```python
from build123d import *

# Parameters (mm, degrees)
SKETCH1_R                                       = 1.6
BASE_FLANGE1_DEPTH                              = 3
EDGE_FLANGE1_START                              = -44
EDGE_FLANGE1_DEPTH                              = 10.5
EDGE_FLANGE1_START_2                            = 33.5
EDGE_FLANGE1_2_DEPTH                            = 10.5
EDGE_FLANGE1_START_3                            = -35
EDGE_FLANGE1_3_DEPTH                            = 1.5
EDGE_FLANGE1_4_DEPTH                            = 1.5
EDGE_FLANGE1_START_4                            = -45.5
EDGE_FLANGE1_5_OUTLINE_W                        = 1.2366
EDGE_FLANGE1_5_OUTLINE_H                        = 3
EDGE_FLANGE1_5_DEPTH                            = 1.5
EDGE_FLANGE1_START_5                            = 44
EDGE_FLANGE1_6_OUTLINE_W                        = 1.2366
EDGE_FLANGE1_6_OUTLINE_H                        = 3
EDGE_FLANGE1_6_DEPTH                            = 1.5
EDGE_FLANGE1_7_DEPTH                            = 9
EDGE_FLANGE1_START_6                            = 35
EDGE_FLANGE1_8_DEPTH                            = 9
CUT_EXTRUDE2_DEPTH                              = 108.796103826
CUT_EXTRUDE2_DEPTH_BACK                         = 108.796103826
SKETCH27_R                                      = 1.6
SKETCH29_R                                      = 1.6
CUT_EXTRUDE4_DEPTH                              = 69.614867194
SKETCH40_W                                      = 1.2366
SKETCH40_H                                      = 2.5
CUT_EXTRUDE5_DEPTH                              = 69.614867194
CSK_FOR_M3_FLAT_HEAD_MACHINE_SCREW1_D           = 3.4
CSK_FOR_M3_FLAT_HEAD_MACHINE_SCREW1_CSINK_D     = 6.3
CSK_FOR_M3_FLAT_HEAD_MACHINE_SCREW1_CSINK_ANGLE = 90


# Read off the part's stored shape, not the designer's step: Edge-Flange1
# Sheet-metal steps are written as plain solids
with BuildPart() as part:
    # Sketch1 → Base-Flange1 (new body)
    with BuildSketch(Plane(origin=(0, 0, 0), x_dir=(1, 0, 0), z_dir=(0, 1, 0))):
        Polygon((-10, 25), (-35, 48), (-44, 48), (-44, 44), (-48, 44), (-48, 35), (-25, 10), (-25, -10), (-48, -35), (-48, -44), (-44, -44), (-44, -48), (-35, -48), (-10, -25), (10, -25), (35, -48), (44, -48), (44, -44), (48, -44), (48, -35), (25, -10), (25, 10), (48, 35), (48, 44), (44, 44), (44, 48), (35, 48), (10, 25), align=None)
        with Locations(Location((-22.000213283, 22.000213283, 0), (0, 0, 270))):
            Circle(SKETCH1_R, mode=Mode.SUBTRACT)
        with Locations(Location((22.000213283, 22.000213283, 0), (0, 0, 270))):
            Circle(SKETCH1_R, mode=Mode.SUBTRACT)
        with Locations(Location((22.000213283, -22.000213283, 0), (0, 0, 270))):
            Circle(SKETCH1_R, mode=Mode.SUBTRACT)
        with Locations(Location((-22.000213283, -22.000213283, 0), (0, 0, 270))):
            Circle(SKETCH1_R, mode=Mode.SUBTRACT)
    extrude(amount=-BASE_FLANGE1_DEPTH)

    # Edge-Flange1 outline → Edge-Flange1 (cut)
    with BuildSketch(Plane.XY.offset(EDGE_FLANGE1_START)):
        with BuildLine():
            ThreePointArc((-47.926677222, -3), (-46.630867001, -0.845704021), (-44.2634, 0))
            Line((-44.2634, 0), (-48, 0))
            Line((-48, 0), (-48, -3))
            Line((-48, -3), (-47.926677222, -3))
        make_face()
        with BuildLine():
            Line((48, 0), (44.2634, 0))
            ThreePointArc((44.2634, 0), (46.630867001, -0.845704021), (47.926677222, -3))
            Line((47.926677222, -3), (48, -3))
            Line((48, -3), (48, 0))
        make_face()
    extrude(amount=EDGE_FLANGE1_DEPTH, mode=Mode.SUBTRACT)

    # Edge-Flange1 2 outline → Edge-Flange1 2 (cut)
    with BuildSketch(Plane.XY.offset(EDGE_FLANGE1_START_2)):
        with BuildLine():
            ThreePointArc((-47.926677222, -3), (-46.630867001, -0.845704021), (-44.2634, 0))
            Line((-44.2634, 0), (-48, 0))
            Line((-48, 0), (-48, -3))
            Line((-48, -3), (-47.926677222, -3))
        make_face()
        with BuildLine():
            Line((48, 0), (44.2634, 0))
            ThreePointArc((44.2634, 0), (46.630867001, -0.845704021), (47.926677222, -3))
            Line((47.926677222, -3), (48, -3))
            Line((48, -3), (48, 0))
        make_face()
    extrude(amount=EDGE_FLANGE1_2_DEPTH, mode=Mode.SUBTRACT)

    # Edge-Flange1 3 outline → Edge-Flange1 3 (cut)
    with BuildSketch(Plane.XY.offset(EDGE_FLANGE1_START_3)):
        with BuildLine():
            Line((-42.7634, -3), (-42.7634, 0))
            Line((-42.7634, 0), (-44.2634, 0))
            ThreePointArc((-44.2634, 0), (-46.630867001, -0.845704021), (-47.926677222, -3))
            Line((-47.926677222, -3), (-42.7634, -3))
        make_face()
        with BuildLine():
            Line((42.7634, 0), (42.7634, -3))
            Line((42.7634, -3), (47.926677222, -3))
            ThreePointArc((47.926677222, -3), (46.630867001, -0.845704021), (44.2634, 0))
            Line((44.2634, 0), (42.7634, 0))
        make_face()
    extrude(amount=EDGE_FLANGE1_3_DEPTH, mode=Mode.SUBTRACT)

    # Edge-Flange1 4 outline → Edge-Flange1 4 (cut)
    with BuildSketch(Plane.XY.offset(EDGE_FLANGE1_START_2)):
        with BuildLine():
            Line((-42.7634, -3), (-42.7634, 0))
            Line((-42.7634, 0), (-44.2634, 0))
            ThreePointArc((-44.2634, 0), (-46.630867001, -0.845704021), (-47.926677222, -3))
            Line((-47.926677222, -3), (-42.7634, -3))
        make_face()
        with BuildLine():
            Line((42.7634, 0), (42.7634, -3))
            Line((42.7634, -3), (47.926677222, -3))
            ThreePointArc((47.926677222, -3), (46.630867001, -0.845704021), (44.2634, 0))
            Line((44.2634, 0), (42.7634, 0))
        make_face()
    extrude(amount=EDGE_FLANGE1_4_DEPTH, mode=Mode.SUBTRACT)

    # Edge-Flange1 5 outline → Edge-Flange1 5 (cut)
    with BuildSketch(Plane.XY.offset(EDGE_FLANGE1_START_4)):
        with Locations((-43.3817, -1.5)):
            Rectangle(EDGE_FLANGE1_5_OUTLINE_W, EDGE_FLANGE1_5_OUTLINE_H)
        with Locations((43.3817, -1.5)):
            Rectangle(EDGE_FLANGE1_5_OUTLINE_W, EDGE_FLANGE1_5_OUTLINE_H)
    extrude(amount=EDGE_FLANGE1_5_DEPTH, mode=Mode.SUBTRACT)

    # Edge-Flange1 6 outline → Edge-Flange1 6 (cut)
    with BuildSketch(Plane.XY.offset(EDGE_FLANGE1_START_5)):
        with Locations((-43.3817, -1.5)):
            Rectangle(EDGE_FLANGE1_6_OUTLINE_W, EDGE_FLANGE1_6_OUTLINE_H)
        with Locations((43.3817, -1.5)):
            Rectangle(EDGE_FLANGE1_6_OUTLINE_W, EDGE_FLANGE1_6_OUTLINE_H)
    extrude(amount=EDGE_FLANGE1_6_DEPTH, mode=Mode.SUBTRACT)

    # Edge-Flange1 7 outline → Edge-Flange1 7 (add)
    with BuildSketch(Plane.XY.offset(EDGE_FLANGE1_START)):
        with BuildLine():
            ThreePointArc((-45, -3.7366), (-44.784254855, -3.215745145), (-44.2634, -3))
            Line((-44.2634, -3), (-47.926677222, -3))
            ThreePointArc((-47.926677222, -3), (-47.981624121, -3.36647982), (-48, -3.7366))
            Line((-48, -3.7366), (-48, -10))
            Line((-48, -10), (-45, -10))
            Line((-45, -10), (-45, -3.7366))
        make_face()
        with BuildLine():
            Line((47.926677222, -3), (44.2634, -3))
            ThreePointArc((44.2634, -3), (44.784254855, -3.215745145), (45, -3.7366))
            Line((45, -3.7366), (45, -10))
            Line((45, -10), (48, -10))
            Line((48, -10), (48, -3.7366))
            ThreePointArc((48, -3.7366), (47.981624121, -3.36647982), (47.926677222, -3))
        make_face()
    extrude(amount=EDGE_FLANGE1_7_DEPTH)

    # Edge-Flange1 8 outline → Edge-Flange1 8 (add)
    with BuildSketch(Plane.XY.offset(EDGE_FLANGE1_START_6)):
        with BuildLine():
            ThreePointArc((-45, -3.7366), (-44.784254855, -3.215745145), (-44.2634, -3))
            Line((-44.2634, -3), (-47.926677222, -3))
            ThreePointArc((-47.926677222, -3), (-47.981624121, -3.36647982), (-48, -3.7366))
            Line((-48, -3.7366), (-48, -10))
            Line((-48, -10), (-45, -10))
            Line((-45, -10), (-45, -3.7366))
        make_face()
        with BuildLine():
            Line((47.926677222, -3), (44.2634, -3))
            ThreePointArc((44.2634, -3), (44.784254855, -3.215745145), (45, -3.7366))
            Line((45, -3.7366), (45, -10))
            Line((45, -10), (48, -10))
            Line((48, -10), (48, -3.7366))
            ThreePointArc((48, -3.7366), (47.981624121, -3.36647982), (47.926677222, -3))
        make_face()
    extrude(amount=EDGE_FLANGE1_8_DEPTH)

    # Sketch27 → Cut-Extrude2 (cut, two sides: drawn at the far end of the back side and taken through both)
    with BuildSketch(Plane.ZY.offset(48).offset(-CUT_EXTRUDE2_DEPTH_BACK)):
        with Locations(Location((39.5, -6.8683, 0), (0, 0, 270))):
            Circle(SKETCH27_R)
        with Locations(Location((-39.5, -6.8683, 0), (0, 0, 270))):
            Circle(SKETCH27_R)
    extrude(amount=CUT_EXTRUDE2_DEPTH + CUT_EXTRUDE2_DEPTH_BACK, mode=Mode.SUBTRACT)

    # Sketch29 → Cut-Extrude4 (cut, through all)
    with BuildSketch(Plane(origin=(0, 0, 0), x_dir=(1, 0, 0), z_dir=(0, 1, 0))):
        with Locations(Location((-36.2, 42.85, 0), (0, 0, 270))):
            Circle(SKETCH29_R)
        with Locations(Location((37.5, 42.85, 0), (0, 0, 270))):
            Circle(SKETCH29_R)
        with Locations(Location((40, -42.85, 0), (0, 0, 270))):
            Circle(SKETCH29_R)
        with Locations(Location((-40, -42.85, 0), (0, 0, 270))):
            Circle(SKETCH29_R)
    extrude(amount=-CUT_EXTRUDE4_DEPTH, mode=Mode.SUBTRACT)

    # Sketch40 → Cut-Extrude5 (cut, through all)
    with BuildSketch(Plane(origin=(0, 0, 0), x_dir=(1, 0, 0), z_dir=(0, 1, 0))):
        Polygon((-42.7634, 35), (-25, 17.2366), (-25, 10), (-46.62, 33.5), (-42.7634, 33.5), align=None)
        with Locations((-43.3817, 46.75)):
            Rectangle(SKETCH40_W, SKETCH40_H)
        Polygon((42.7634, 33.5), (42.7634, 35), (25, 17.2366), (25, 10), (46.62, 33.5), align=None)
        with Locations((43.3817, 46.75)):
            Rectangle(SKETCH40_W, SKETCH40_H)
        Polygon((42.7634, -35), (25, -17.2366), (25, -10), (46.62, -33.5), (42.7634, -33.5), align=None)
        with Locations((43.3817, -46.75)):
            Rectangle(SKETCH40_W, SKETCH40_H)
        Polygon((-42.7634, -33.5), (-42.7634, -35), (-25, -17.2366), (-25, -10), (-46.62, -33.5), align=None)
        with Locations((-43.3817, -46.75)):
            Rectangle(SKETCH40_W, SKETCH40_H)
    extrude(amount=-CUT_EXTRUDE5_DEPTH, mode=Mode.SUBTRACT)

    # CSK for M3 Flat Head Machine Screw1 (through all)
    with Locations(Plane(origin=(0, 0, 0), x_dir=(1, 0, 0), z_dir=(0, 1, 0))):
        with Locations((-22.000213283, 22.000213283), (22.000213283, 22.000213283), (22.000213283, -22.000213283), (-22.000213283, -22.000213283)):
            CounterSinkHole(CSK_FOR_M3_FLAT_HEAD_MACHINE_SCREW1_D / 2, CSK_FOR_M3_FLAT_HEAD_MACHINE_SCREW1_CSINK_D / 2, counter_sink_angle=CSK_FOR_M3_FLAT_HEAD_MACHINE_SCREW1_CSINK_ANGLE)


solid = part.part
```
The listing builds one solid part. Answer for the finished solid, in the listing's coordinates (mm). A direction names the side the tool comes from. Coordinates: 2 decimals unless noted, no trailing zeros. Loops run counter-clockwise (first coordinate to the right, second up) from the corner with the lowest first, then second, coordinate; pieces in that order, holes last. Notation, with made-up numbers: (1.25, 44.5) -> (40.25, 44.5) arc R21 ccw to (40.25, 71.5) -> close; hole circle Ø2 at (-10.5, 31.5). An arc over 180 degrees is marked (long way). Use one line per item in the form item = value. Start each with the question number.
Item 1: The part is cut by section B-B on x = -40. Determine the outline of the cut face in (y, z), then the cut area to 3 significant figures.
Item 2: The mould has two halves that part along Z. Classify faces 1 (the face through (34.006, -1.479, -26.243)), 2 (the face through (-46, -5, 44)), 3 (the face through (45, -8, -41)): released by +Z, released by -Z, zero draft, split by the parting line, or undercut.
Item 3: A tool of negligible diameter and unlimited length cuts with its end or side. For faces 4 (the face through (-42.763, -1, 46)), 5 (the face through (46, -5, -35)), 6 (the face through (-22.325, -1.479, -36.339)), from which of +Z, -Z, +X, -X, +Y, -Y can it reach the whole face along a straight path? Write none if from no direction.
Item 4: Consider L1, parallel to X at y = -2, z = -43.5; L2, parallel to X at y = -1.45, z = 42.85; L3, parallel to X at y = -1.5, z = 20.5. Determine where each line is inside the solid, lowest interval first. Write a range as [from, to].
Item 5: The part is cut by section C-C on x = -27. Determine the outline of the cut face in (y, z).
Item 6: Flat-ended cylindrical pins translate along their axes: pin 1 Ø1.6 at (x, y) = (-46.5, -7) entering from -Z; pin 2 Ø5 at (y, z) = (-5, -29) entering from +X; pin 3 Ø0.9 at (y, z) = (-1, 45.5) entering from +X. Find the tip coordinate at first contact, or state that the pin passes through.
Item 7: The part is cut by section A-A on z = 39.5. Determine the outline of the cut face in (x, y).
Item 8: The part is cut by section D-D on z = 10. Determine the outline of the cut face in (x, y).
Answer key:
q1.outline = (-3, -48) -> (0, -48) -> (0, -32.24) -> (-3, -32.24) -> close; (-3, 32.24) -> (0, 32.24) -> (0, 41.25) -> (-3, 41.25) -> close; (-3, 44.45) -> (0, 44.45) -> (0, 48) -> (-3, 48) -> close
q1.area = 85.0 mm2
q2.face_1 = undercut
q2.face_2 = released by +Z
q2.face_3 = zero draft
q3.face_4 = +Z, -X, +Y, -Y
q3.face_5 = +X, +Y, -Y
q3.face_6 = -Z, +Y, -Y
q4.L1 = [-47.57, -37.66], [-34.74, -30.11], [30.11, 36.04], [38.96, 47.57]
q4.L2 = [-47.22, -41.6], [-38.4, -29.4], [29.4, 38.4], [41.6, 47.22]
q4.L3 = [-28.26, -22.8], [-21.2, 21.2], [22.8, 28.26]
q5.outline = (-3, -40.64) -> (0, -40.64) -> (0, -19.24) -> (-3, -19.24) -> close; (-3, 19.24) -> (0, 19.24) -> (0, 40.64) -> (-3, 40.64) -> close
q6.pin_1 = -44
q6.pin_2 = 38.26
q6.pin_3 = 42.76
q7.outline = (-48, -10) -> (-45, -10) -> (-45, -8.47) -> (-48, -8.47) -> close; (-48, -5.27) -> (-45, -5.27) -> (-45, -3.74) arc R0.74 cw to (-44.26, -3) -> (-25.76, -3) -> (-25.76, 0) -> (-44.26, 0) arc R3.74 ccw to (-48, -3.74) -> close; (25.76, -3) -> (44.26, -3) arc R0.74 cw to (45, -3.74) -> (45, -5.27) -> (48, -5.27) -> (48, -3.74) arc R3.74 ccw to (44.26, 0) -> (25.76, 0) -> close; (45, -10) -> (48, -10) -> (48, -8.47) -> (45, -8.47) -> close
q8.outline = (-25, -3) -> (25, -3) -> (25, 0) -> (-25, 0) -> close
